Geometry: final body of the model. Coordinates: model frame, mm. A direction names the side the tool comes from. Coordinates: 2 decimals unless noted, no trailing zeros. Order: outer loops, then holes, each group sorted by start corner. A loop starts at its lowest first (then second) coordinate and runs counter-clockwise, first axis right, second up. Notation, with made-up numbers: M 3.25,-1.75 L 52.25,-1.75 A17 ccw 52.25,9.25 Z; hole C 3,29.25 d6. An arc over 180 degrees is marked long. Use CSV: the item, a comma, the result in double quotes. Start each with the question number.
Q1. Access query for faces 1 (the face through (-19, 0, 30)), 2 (the face through (-18.8, 6, 16)), 3 (the face through (-22.753, 1, 32)), 4 (the face through (-18.8, 6, 29.3)), 5 (the face through (-18.7, 6, 15)). Directions: +Z, -Z, +X, -X, +Y, -Y. A direction counts if a zero-diameter tool reaches every point of the face in a straight line with its end or side. Return the directions, or none.
Q2. Ray query, probe 1 along Y at (x, z) = (-19, 35); probe 2 along Z at (x, y) = (-22, -9); probe 3 along Z at (x, y) = (-16.25, 5.25). Return the intervals inside material, ascending.
Q3. Mould query, pull axis Z, two halves, no side actions, for faces 6 (the face through (-19, -5, 60)), 7 (the face through (-18.7, 6, 28.3)), 8 (the face through (-19, -6, 59)). Classes: +Z half, -Z half, draft (parallel to the pull), parting line (faces both ways), or undercut.
Q4. Section query C-C, the plane z = 40.5. Output: boundary loops of the cut face in (x, y).
Q5. First-contact query: P1, Ø1.5, axis at x = -18.5, z = 50, coming from the +Y side; P2, Ø2.5, axis at x = -19.5, z = 40.5, coming from the -Y side; P3, Ø3, axis at y = 6, z = 51.5, coming from the +X side; P4, Ø2, axis at x = -21, y = -2, coming from the -Z side. Flat tips, straight axial feed; report the tip coordinate or a pass-through.
Q6. Section query A-A, the plane y = 7. Output: boundary loops of the cut face in (x, z), and give its area (3 significant figures).
Q7. Section query B-B, the plane x = -17.25. Output: boundary loops of the cut face in (y, z).
Q8. Section query D-D, the plane y = -7.5. Output: boundary loops of the cut face in (x, z), and give its area (3 significant figures).
from build123d import *

# Parameters (mm, degrees)
F1_DEPTH = 3
F3_DEPTH = 6
F2_W     = 8
F2_H     = 1
F4_DEPTH = 15


with BuildPart() as f1:
    # F0 (on Front) → F1 (new body)
    with BuildSketch(Plane.XZ):
        with BuildLine():
            ThreePointArc((-22.7528382093, 28.0764238795), (-18.7528382093, 29.3), (-14.7528382093, 28.0764238795))
            Line((-14.7528382093, 28.0764238795), (-14.7528382093, 60))
            Line((-14.7528382093, 60), (-22.7528382093, 60))
            Line((-22.7528382093, 60), (-22.7528382093, 28.0764238795))
        make_face()
        with BuildLine():
            ThreePointArc((-22.7528382093, 16.2235761205), (-18.7528382093, 15), (-14.7528382093, 16.2235761205))
            Line((-14.7528382093, 16.2235761205), (-14.7528382093, 28.0764238795))
            ThreePointArc((-14.7528382093, 28.0764238795), (-18.7528382093, 29.3), (-22.7528382093, 28.0764238795))
            Line((-22.7528382093, 28.0764238795), (-22.7528382093, 16.2235761205))
        make_face()
        with BuildLine():
            Line((-22.7528382093, 0), (-14.7528382093, 0))
            Line((-14.7528382093, 0), (-14.7528382093, 16.2235761205))
            ThreePointArc((-14.7528382093, 16.2235761205), (-18.7528382093, 15), (-22.7528382093, 16.2235761205))
            Line((-22.7528382093, 16.2235761205), (-22.7528382093, 0))
        make_face()
    extrude(amount=-F1_DEPTH)

    # F2 (on face) → F3 (join)
    with BuildSketch(Plane(origin=(0, 3, 0), x_dir=(-1, 0, 0), z_dir=(0, 1, 0))):
        with BuildLine():
            ThreePointArc((22.7528382093, 28.0764238795), (18.7528382093, 29.3), (14.7528382093, 28.0764238795))
            Line((14.7528382093, 28.0764238795), (14.7528382093, 26.8214558758))
            ThreePointArc((14.7528382093, 26.8214558758), (18.7528382093, 28.3), (22.7528382093, 26.8214558758))
            Line((22.7528382093, 26.8214558758), (22.7528382093, 28.0764238795))
        make_face()
        with BuildLine():
            Line((14.7528382093, 17.4785441242), (14.7528382093, 16.2235761205))
            ThreePointArc((14.7528382093, 16.2235761205), (18.7528382093, 15), (22.7528382093, 16.2235761205))
            Line((22.7528382093, 16.2235761205), (22.7528382093, 17.4785441242))
            ThreePointArc((22.7528382093, 17.4785441242), (18.7528382093, 16), (14.7528382093, 17.4785441242))
        make_face()
    extrude(amount=F3_DEPTH)

    # F2 (on face) → F4 (join)
    with BuildSketch(Plane(origin=(0, 3, 0), x_dir=(-1, 0, 0), z_dir=(0, 1, 0))):
        with Locations((18.7528382093, 59.5)):
            Rectangle(F2_W, F2_H)
    extrude(amount=-F4_DEPTH)


solid = f1.part
Responses:
1,face 1,"-Z, +X, -X, -Y"
1,face 2,"+Y"
1,face 3,"+Z, -Z, -X, +Y, -Y"
1,face 4,"+Z, +Y"
1,face 5,"-Z, +Y"
2,probe 1,"y = 0 to 3"
2,probe 2,"z = 59 to 60"
2,probe 3,"z = 15.45 to 16.53, 27.77 to 28.85"
3,face 6,"+Z half"
3,face 7,"undercut"
3,face 8,"-Z half"
4,outline,"M -22.75,0 L -14.75,0 L -14.75,3 L -22.75,3 Z"
5,P1,"stops at y = 3"
5,P2,"stops at y = 0"
5,P3,"passes through"
5,P4,"stops at z = 59"
6,outline,"M -22.75,16.22 A7.15 ccw -14.75,16.22 L -14.75,17.48 A6.15 cw -22.75,17.48 Z; M -22.75,26.82 A6.15 cw -14.75,26.82 L -14.75,28.08 A7.15 ccw -22.75,28.08 Z"
6,area,"17.2 mm²"
7,outline,"M -12,59 L 0,59 L 0,0 L 3,0 L 3,15.16 L 9,15.16 L 9,16.19 L 3,16.19 L 3,28.11 L 9,28.11 L 9,29.14 L 3,29.14 L 3,60 L -12,60 Z"
8,outline,"M -22.75,59 L -14.75,59 L -14.75,60 L -22.75,60 Z"
8,area,"8.00 mm²"
